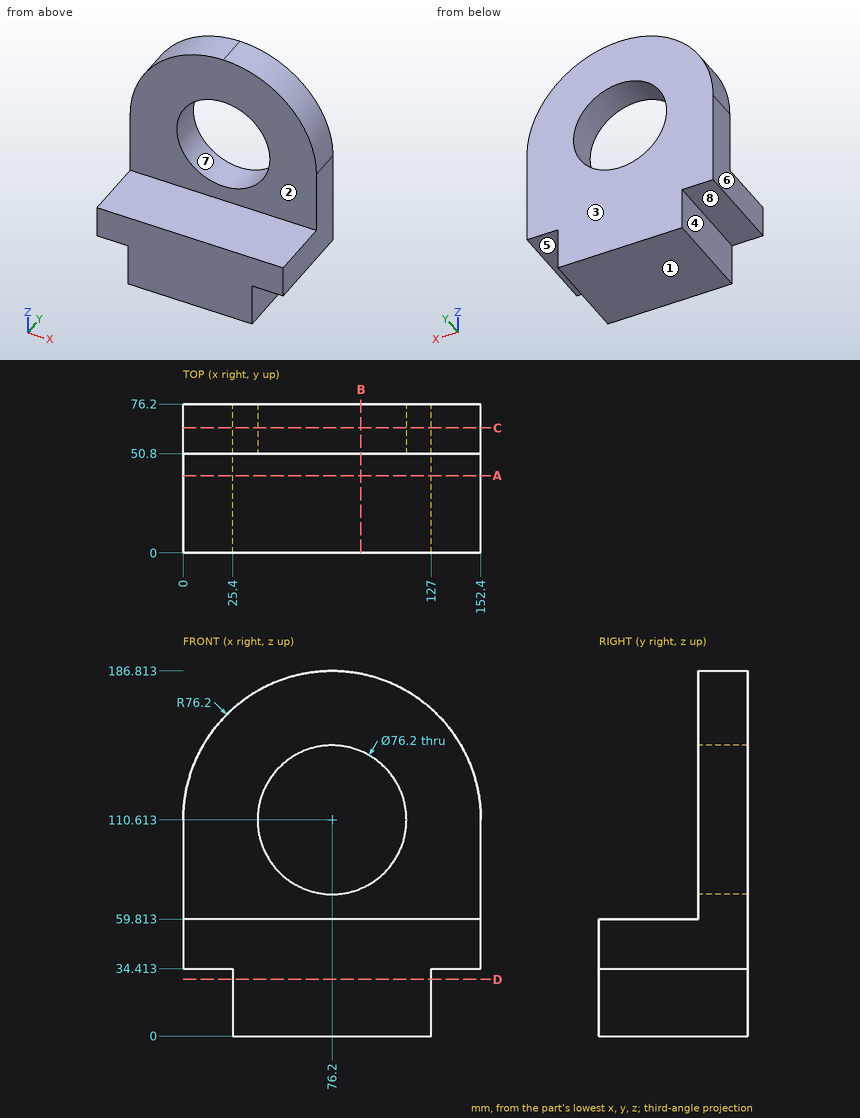
Can you work these out from the drawing? Everything is in mm from the part's minimum corner. A direction names the side the tool comes from. Round coordinates to 2 decimals unless told otherwise and drop trailing zeros. Write each loop counter-clockwise with the first axis right and the second up, starting at its lowest first coordinate (ties: lowest second). Pieces come first, ordered by that corner, then holes.
1. Suppose I cut it at D-D (z = 29). List the corners of the cut face in (x, y) for me, and give its area (3 significant figures).
2. Suppose I cut it at B-B (x = 91). List the corners of the cut face in (y, z) for me (3 decimals), and give its area (3 significant figures).
3. Will these pins go through, and if not, where does the flat tip stop? pin 1 Ø1 at (x, y) = (21.5, 48.5) entering from -Z; pin 2 Ø6 at (x, y) = (104, 34.5) entering from +Z; pin 3 Ø17 at (y, z) = (30, 12) entering from -X.
4. I need wall thicknesses on L1, parallel to Z at x = 76.2, y = 70; L2, parallel to Y at x = 142, z = 122; L3, parallel to X at y = 27, z = 9. Which ranges of each line are inside material? Lowest first, please.
5. For the marked faces 1, 2, 3, 4 and 5, which set-ups out of +Z, -Z, +X, -X, +Y, -Y let a thin tool reach every point of the face, with its end or its side?
6. If we mould it in two halves opening along X, with no side actions, what happens to the marked faces 6, 7 and 8? For each: released by +X, released by -X, zero draft, split by the parting line, or undercut.
7. Suppose I cut it at A-A (y = 39.5). List the corners of the cut face in (x, z) for me.
8. Suppose I cut it at C-C (y = 64). List the corners of the cut face in (x, z) for me, and give its area (3 significant figures).
Answer sheet:
1. outline: (25.4, 0) - (127, 0) - (127, 76.2) - (25.4, 76.2) - close
1. area: 7,740 mm2
2. outline: (0, 0) - (76.2, 0) - (76.2, 75.505) - (50.8, 75.505) - (50.8, 59.813) - (0, 59.813) - close; (50.8, 145.721) - (76.2, 145.721) - (76.2, 185.362) - (50.8, 185.362) - close
2. area: 5,960 mm2
3. pin 1: stops at z = 34.41
3. pin 2: stops at z = 59.81
3. pin 3: stops at x = 25.4
4. L1: z = 0 to 72.51, 148.71 to 186.81
4. L2: y = 50.8 to 76.2
4. L3: x = 25.4 to 127
5. face 1: -Z, +X, -X, +Y, -Y
5. face 2: +Z, +X, -X, -Y
5. face 3: +Z, -Z, +X, -X, +Y
5. face 4: -Z, -X, +Y, -Y
5. face 5: -Z, +X, +Y, -Y
6. face 6: released by -X
6. face 7: undercut
6. face 8: zero draft
7. outline: (0, 34.41) - (25.4, 34.41) - (25.4, 0) - (127, 0) - (127, 34.41) - (152.4, 34.41) - (152.4, 59.81) - (0, 59.81) - close
8. outline: (0, 34.41) - (25.4, 34.41) - (25.4, 0) - (127, 0) - (127, 34.41) - (152.4, 34.41) - (152.4, 110.61) arc R76.2 ccw to (76.2, 186.81) arc R76.2 ccw to (0, 110.61) - close; hole circle Ø76.2 at (76.2, 110.61)
8. area: 19,700 mm2
